```python
from build123d import *

# Parameters (mm, degrees)
BOSS_EXTRUDE1_DEPTH      = 140
BOSS_EXTRUDE1_DEPTH_BACK = 140
LPATTERN2_COUNT          = 5
LPATTERN2_PITCH          = 60
CHAMFER1_SIZE            = 0.5
CUT_EXTRUDE1_DEPTH       = 1
CUT_EXTRUDE1_DEPTH_BACK  = 19


with BuildPart() as part:
    # Sketch3 → Boss-Extrude1 (new body, two sides)
    with BuildSketch(Plane.XY) as boss_extrude1_sk:
        with BuildLine():
            Line((3, 9), (-3, 9))
            Line((-3, 9), (-7.160036564, 9))
            Line((-7.160036564, 9), (-7.767930373, 8.392105714))
            ThreePointArc((-7.767930373, 8.392105714), (-8.344874488, 7.264307267), (-9.472673258, 6.687363783))
            Line((-9.472673258, 6.687363783), (-10, 6.160037041))
            Line((-10, 6.160037041), (-10, 4.82918644))
            Line((-10, 4.82918644), (-9.472673258, 4.314376637))
            ThreePointArc((-9.472673258, 4.314376637), (-8.341068744, 3.731631743), (-7.767930373, 2.595131504))
            Line((-7.767930373, 2.595131504), (-6.550048828, 1.379235268))
            Line((-6.550048828, 1.379235268), (-6.550048828, -1.550048828))
            Line((-6.550048828, -1.550048828), (-10, -4.999922752))
            Line((-10, -4.999922752), (-10, -8))
            Line((-10, -8), (-9, -9))
            Line((-9, -9), (0, -9))
            Line((0, -9), (9, -9))
            Line((9, -9), (10, -8))
            Line((10, -8), (10, -4.999922752))
            Line((10, -4.999922752), (6.550048828, -1.550048828))
            Line((6.550048828, -1.550048828), (6.550048828, 1.379235268))
            Line((6.550048828, 1.379235268), (7.767930373, 2.595131504))
            ThreePointArc((7.767930373, 2.595131504), (8.341068744, 3.731631743), (9.472673258, 4.314376637))
            Line((9.472673258, 4.314376637), (10, 4.82918644))
            Line((10, 4.82918644), (10, 6.160037041))
            Line((10, 6.160037041), (9.472673258, 6.687363783))
            ThreePointArc((9.472673258, 6.687363783), (8.344874488, 7.264307267), (7.767930373, 8.392105714))
            Line((7.767930373, 8.392105714), (7.160036564, 9))
            Line((7.160036564, 9), (3, 9))
        make_face()
    extrude(amount=BOSS_EXTRUDE1_DEPTH)
    extrude(boss_extrude1_sk.sketch, amount=-BOSS_EXTRUDE1_DEPTH_BACK)

    # Sketch4 → Cut-Revolve1 (revolve, cut)
    with BuildSketch(Plane(origin=(0, 0, 0), x_dir=(0, 0, -1), z_dir=(1, 0, 0))):
        Polygon((-115.25, 9), (-120, 9), (-120, -9), (-117, -9), (-117, 0.5), (-115.25, 0.5), align=None)
    cut_revolve1 = revolve(axis=Axis((0, 9, 120), (0, -1, 0)), mode=Mode.SUBTRACT)

    # LPattern2: Cut-Revolve1 ×5
    with Locations(*[(0, 0, -i * LPATTERN2_PITCH) for i in range(1, LPATTERN2_COUNT)]):
        add(cut_revolve1, mode=Mode.SUBTRACT)

    # Chamfer1
    chamfer1_edges = [part.edges().sort_by_distance(p)[0] for p in [
        (-6.550048828, -0.08540678, 140),
        (-8.275024414, -3.27498579, 140),
        (-10, -6.499961376, 140),
        (-9.5, -8.5, 140),
        (0, -9, 140),
        (9.5, -8.5, 140),
        (10, -6.499961376, 140),
        (8.275024414, -3.27498579, 140),
        (6.550048828, -0.08540678, 140),
        (-8.341068744, 3.731631743, 140),
        (7.158989601, 1.987183386, 140),
        (8.341068744, 3.731631743, 140),
        (9.736336629, 4.571781538, 140),
        (-9.736336629, 4.571781538, -140),
        (-10, 5.49461174, -140),
        (10, 5.49461174, 140),
        (-9.736336629, 6.423700412, -140),
        (-7.463983469, 8.696052857, -140),
        (0, 9, -140),
        (7.463983469, 8.696052857, -140),
        (9.736336629, 6.423700412, -140),
        (10, 5.49461174, -140),
        (9.736336629, 6.423700412, 140),
        (9.736336629, 4.571781538, -140),
        (7.158989601, 1.987183386, -140),
        (6.550048828, -0.08540678, -140),
        (8.275024414, -3.27498579, -140),
        (10, -6.499961376, -140),
        (9.5, -8.5, -140),
        (0, -9, -140),
        (8.344874488, 7.264307267, 140),
        (-9.5, -8.5, -140),
        (-10, -6.499961376, -140),
        (-8.275024414, -3.27498579, -140),
        (-6.550048828, -0.08540678, -140),
        (-7.158989601, 1.987183386, -140),
        (-8.341068744, 3.731631743, -140),
        (-8.344874488, 7.264307267, -140),
        (8.344874488, 7.264307267, -140),
        (8.341068744, 3.731631743, -140),
        (7.463983469, 8.696052857, 140),
        (0, 9, 140),
        (-7.463983469, 8.696052857, 140),
        (-8.344874488, 7.264307267, 140),
        (-7.158989601, 1.987183386, 140),
        (-9.736336629, 6.423700412, 140),
        (-10, 5.49461174, 140),
        (-9.736336629, 4.571781538, 140),
    ]]
    chamfer(chamfer1_edges, length=CHAMFER1_SIZE)

    # Sketch7 → Cut-Extrude1 (cut, two sides)
    with BuildSketch(Plane.XZ.offset(9)) as cut_extrude1_sk:
        Polygon((563.970585521, -126.7), (15.689992686, -126.7), (-26.160878802, -126.7), (-574.441471637, -126.7), (-574.441471637, -1223.26118567), (563.970585521, -1223.26118567), align=None)
    extrude(amount=CUT_EXTRUDE1_DEPTH, mode=Mode.SUBTRACT)
    extrude(cut_extrude1_sk.sketch, amount=-CUT_EXTRUDE1_DEPTH_BACK, mode=Mode.SUBTRACT)


solid = part.part
```
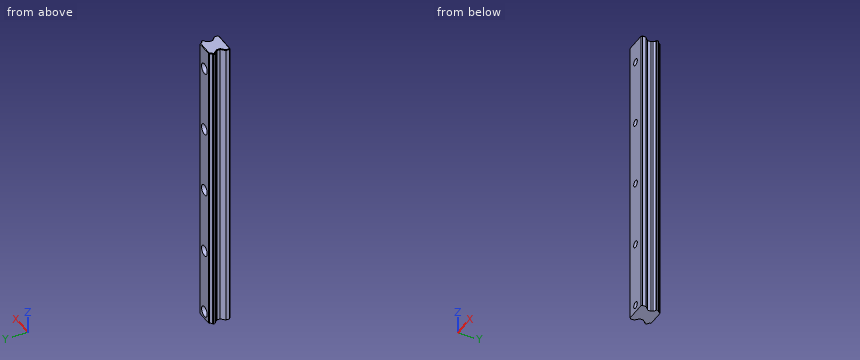
Input: part model. Units: mm. Frame: model coordinates. Give positions to 0.01 mm unless a question says otherwise; leave off trailing zeros. One line per question, with ' | ' between items.
1) Ray query, L1, parallel to Y at x = -6.75, z = -85.5; L2, parallel to X at y = -4.25, z = 120; L3, parallel to X at y = -3.5, z = 0. Return the intervals inside material, ascending.
Filled in:
L1: y = -9 to -1.75, 1.58 to 9 | L2: x = -9.25 to -3, 3 to 9.25 | L3: x = -8.5 to -3, 3 to 8.5
2) Contact query for flat-ended pins moving along their axis: P1, Ø11, axis at x = 0, z = -120, coming from the -Y side; P2, Ø3, axis at x = -0.5, z = 118.5, coming from the +Y side; P3, Ø2.5, axis at y = -0.5, z = -19, coming from the +X side; P4, Ø1, axis at y = 0, z = 58, coming from the -X side. Output: stop coordinate, or through.
Filled in:
P1: stops at y = -9 | P2: stops at y = 0.5 | P3: stops at x = 6.75 | P4: stops at x = -6.55
3) Section B-B on x = 0. State how many separate pieces and enclosed holes the cut face has, and give its area (3 significant figures).
Filled in:
separate pieces: 6 | enclosed holes: 0 | area: 4,110 mm2
